The listing builds one solid part. Answer for the finished solid, in the listing's coordinates (mm). Face numbers are marked on the shaded views. A direction names the side the tool comes from. Coordinates: 2 decimals unless noted, no trailing zeros. Order: outer loops, then holes, each group sorted by start corner. A loop starts at its lowest first (then second) coordinate and runs counter-clockwise, first axis right, second up. Notation, with made-up numbers: (7.5, 83) -> (13.5, 83) arc R25 ccw to (13.5, 122) -> close; hole circle Ø9 at (-1.75, 14.5). An arc over 180 degrees is marked (long way). Write item = value, one per line. Start each with the question number.
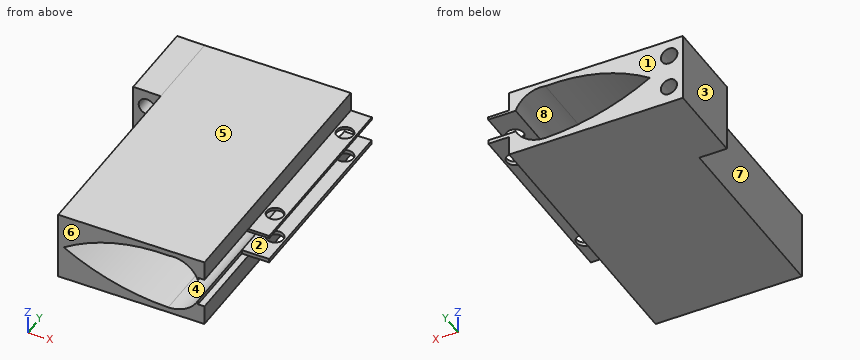
```python
from build123d import *

# Parameters (mm, degrees)
SKETCH1_W           = 67.320921889
SKETCH1_H           = 31.744824956
BOSS_EXTRUDE1_DEPTH = 127
BOSS_EXTRUDE2_DEPTH = 38.1
SKETCH3_R           = 3.798675559
CUT_EXTRUDE1_DEPTH  = 53.34
SKETCH4_R           = 3.713025355
CUT_EXTRUDE2_DEPTH  = 72.898
CUT_EXTRUDE3_DEPTH  = 177.8
CUT_EXTRUDE4_DEPTH  = 140.752657
SKETCH7_W           = 12.598265338
SKETCH7_H           = 1.777860749
BOSS_EXTRUDE3_DEPTH = 88.936657
SKETCH8_W           = 12.621827424
SKETCH8_H           = 1.259783395
BOSS_EXTRUDE4_DEPTH = 88.936657
SKETCH9_R           = 3.862443539
CUT_EXTRUDE5_DEPTH  = 31.278657
SKETCH10_R          = 3.842033399
CUT_EXTRUDE6_DEPTH  = 32.548657


with BuildPart() as part:
    # Sketch1 → Boss-Extrude1 (new body)
    with BuildSketch(Plane(origin=(0, 0, 0), x_dir=(1, 0, 0), z_dir=(0, 1, 0))):
        with Locations((33.660460945, -15.872412478)):
            Rectangle(SKETCH1_W, SKETCH1_H)
    extrude(amount=BOSS_EXTRUDE1_DEPTH)

    # Sketch2 → Boss-Extrude2 (add)
    with BuildSketch(Plane(origin=(0, 127, 0), x_dir=(1, 0, 0), z_dir=(0, 1, 0))):
        Polygon((0, 0), (-12.691812955, 0), (-12.691812955, -31.893008725), (0, -31.744824956), align=None)
    extrude(amount=-BOSS_EXTRUDE2_DEPTH)

    # Sketch3 → Cut-Extrude1 (cut)
    with BuildSketch(Plane(origin=(0, 127, 0), x_dir=(1, 0, 0), z_dir=(0, 1, 0))):
        with Locations(Location((-6.345906477, -23.919756544, 0), (0, 0, 270))):
            Circle(SKETCH3_R)
    extrude(amount=-CUT_EXTRUDE1_DEPTH, mode=Mode.SUBTRACT)

    # Sketch4 → Cut-Extrude2 (cut)
    with BuildSketch(Plane(origin=(0, 127, 0), x_dir=(1, 0, 0), z_dir=(0, 1, 0))):
        with Locations(Location((-6.238928802, -8.074927798, 0), (0, 0, 270))):
            Circle(SKETCH4_R)
    extrude(amount=-CUT_EXTRUDE2_DEPTH, mode=Mode.SUBTRACT)

    # Sketch5 → Cut-Extrude3 (cut)
    with BuildSketch(Plane(origin=(0, 127, 0), x_dir=(1, 0, 0), z_dir=(0, 1, 0))):
        with BuildLine():
            ThreePointArc((64.884408785, -12.014730435), (65.337632333, -15.775676375), (64.884408785, -19.536622316))
            ThreePointArc((64.884408785, -19.536622316), (59.764565977, -27.313148833), (50.645455775, -29.191707899))
            ThreePointArc((50.645455775, -29.191707899), (25.520797189, -26.413912497), (2.545998088, -15.872412478))
            ThreePointArc((2.545998088, -15.872412478), (25.757322084, -6.167748294), (50.645455775, -2.489858962))
            ThreePointArc((50.645455775, -2.489858962), (59.21392875, -5.086156005), (64.884408785, -12.014730435))
        make_face()
    extrude(amount=-CUT_EXTRUDE3_DEPTH, mode=Mode.SUBTRACT)

    # Sketch6 → Cut-Extrude4 (cut)
    with BuildSketch(Plane(origin=(0, 127, 0), x_dir=(1, 0, 0), z_dir=(0, 1, 0))):
        Polygon((64.338150371, -15.872412478), (64.338150371, -22.747923603), (67.320921889, -22.747923603), (67.320921889, -9.054734185), (64.338150371, -9.054734185), align=None)
    extrude(amount=-CUT_EXTRUDE4_DEPTH, mode=Mode.SUBTRACT)

    # Sketch7 → Boss-Extrude3 (add)
    with BuildSketch(Plane(origin=(0, 127, 0), x_dir=(1, 0, 0), z_dir=(0, 1, 0))):
        with Locations((70.63728304, -9.94366456)):
            Rectangle(SKETCH7_W, SKETCH7_H)
    extrude(amount=-BOSS_EXTRUDE3_DEPTH)

    # Sketch8 → Boss-Extrude4 (add)
    with BuildSketch(Plane(origin=(0, 127, 0), x_dir=(1, 0, 0), z_dir=(0, 1, 0))):
        with Locations((70.649064083, -22.118031906)):
            Rectangle(SKETCH8_W, SKETCH8_H)
    extrude(amount=-BOSS_EXTRUDE4_DEPTH)

    # Sketch9 → Cut-Extrude5 (cut)
    with BuildSketch(Plane(origin=(0, 0, 9.054734185), x_dir=(-1, 0, 0), z_dir=(0, 0, -1))):
        with Locations((-72.128668799, 112.805210201)):
            Circle(SKETCH9_R)
    extrude(amount=-CUT_EXTRUDE5_DEPTH, mode=Mode.SUBTRACT)

    # Sketch10 → Cut-Extrude6 (cut)
    with BuildSketch(Plane(origin=(0, 0, 9.054734185), x_dir=(-1, 0, 0), z_dir=(0, 0, -1))):
        with Locations((-72.128668799, 52.198950376)):
            Circle(SKETCH10_R)
    extrude(amount=-CUT_EXTRUDE6_DEPTH, mode=Mode.SUBTRACT)


solid = part.part
```
Item 1: Which of the six approach directions +Z, -Z, +X, -X, +Y, -Y give full straight-line access (tool end or side, diameter ignored) to the marked faces 1, 2, 3, 4 and 5?
Item 2: Section D-D, the plane y = 98 is taken. Give the vertices of the cut face in (x, z), then the cut area to 3 significant figures.
Item 3: For a pull along X with two mould halves and no side action, classify the marked faces 6, 7 and 8 as pulls with the +X half, pulls with the -X half, needs draft (parallel to the pull), parting line crosses it, or undercut.
Item 4: Consider probe 1 along Z at (x, y) = (71, 70); probe 2 along X at (y, z) = (75.5, 30.5); probe 3 along X at (y, z) = (101.5, 22.5). Determine where each line is inside the solid, lowest interval first.
Item 5: Section B-B, the plane x = 71 is taken. Give the vertices of the cut face in (y, z).
Item 6: Section C-C, the plane z = 7 is taken. Give the vertices of the cut face in (x, y).
Item 7: Section A-A, the plane x = 47.5 is taken. Give the vertices of the cut face in (y, z).
Item 8: Each of these flat-tipped pins is pushed along its axis until it touches: pin 1 (2.5 mm diameter, centred on x = 66, y = 9.5, fed in from +Z); pin 2 (2.5 mm diameter, centred on y = 68, z = 3.5, fed in from +X); pin 3 (14 mm diameter, centred on x = -8, z = 14, fed in from -Y). Where does it stop, or does it pass through?
A:
q1.face_1 = +Z, -Z, +X, -X, +Y
q1.face_2 = +X, +Y, -Y
q1.face_3 = +Z, -Z, -X, +Y, -Y
q1.face_4 = +Y, -Y
q1.face_5 = +Z, +X, +Y, -Y
q2.outline = (-12.69, 0) -> (67.32, 0) -> (67.32, 9.05) -> (76.94, 9.05) -> (76.94, 10.83) -> (64.34, 10.83) arc R15.38 cw to (50.65, 2.49) arc R101.18 cw to (2.55, 15.87) arc R79.32 cw to (50.65, 29.19) arc R12.16 cw to (64.34, 21.49) -> (76.96, 21.49) -> (76.96, 22.75) -> (67.32, 22.75) -> (67.32, 31.74) -> (0, 31.74) -> (-12.69, 31.89) -> close; hole circle Ø7.6 at (-6.35, 23.92); hole circle Ø7.43 at (-6.24, 8.07)
q2.area = 1,260 mm^2
q3.face_6 = needs draft
q3.face_7 = pulls with the -X half
q3.face_8 = undercut
q4.probe_1 = 9.05 to 10.83, 21.49 to 22.75
q4.probe_2 = 0 to 67.32
q4.probe_3 = -12.69 to -9.87, -2.82 to 14.58, 63.91 to 76.96
q5.outline = (38.06, 9.05) -> (48.53, 9.05) -> (48.53, 10.83) -> (38.06, 10.83) -> close; (38.06, 21.49) -> (48.53, 21.49) -> (48.53, 22.75) -> (38.06, 22.75) -> close; (55.87, 9.05) -> (109.11, 9.05) -> (109.11, 10.83) -> (55.87, 10.83) -> close; (55.87, 21.49) -> (109.11, 21.49) -> (109.11, 22.75) -> (55.87, 22.75) -> close; (116.5, 9.05) -> (127, 9.05) -> (127, 10.83) -> (116.5, 10.83) -> close; (116.5, 21.49) -> (127, 21.49) -> (127, 22.75) -> (116.5, 22.75) -> close
q6.outline = (-12.69, 88.9) -> (-9.79, 88.9) -> (-9.79, 127) -> (-12.69, 127) -> close; (-2.68, 88.9) -> (0, 88.9) -> (0, 0) -> (22.93, 0) -> (22.93, 127) -> (-2.68, 127) -> close; (61.54, 0) -> (67.32, 0) -> (67.32, 127) -> (61.54, 127) -> close
q7.outline = (0, 0) -> (127, 0) -> (127, 2.61) -> (0, 2.61) -> close; (0, 29.29) -> (127, 29.29) -> (127, 31.74) -> (0, 31.74) -> close
q8.pin_1 = 31.74
q8.pin_2 = 67.32
q8.pin_3 = 88.9
